from build123d import *

# Parameters (mm, degrees)
SKETCH1_W           = 40
SKETCH1_H           = 33.75
SKETCH1_R           = 2.5
BOSS_EXTRUDE1_DEPTH = 6.25
SKETCH1_3_W         = 40
SKETCH1_3_H         = 6.25
BOSS_EXTRUDE2_DEPTH = 40
FILLET1_R           = 6.25
FILLET2_R           = 1.25
SKETCH2_R           = 5
CUT_EXTRUDE1_DEPTH  = 40


with BuildPart() as part:
    # Sketch1 → Boss-Extrude1 (new body)
    with BuildSketch(Plane(origin=(0, 0, 0), x_dir=(1, 0, 0), z_dir=(0, 1, 0))):
        with Locations((20, 16.875)):
            Rectangle(SKETCH1_W, SKETCH1_H)
        with Locations(Location((10, 15, 0), (0, 0, 270))):
            Circle(SKETCH1_R, mode=Mode.SUBTRACT)
        with Locations(Location((30, 15, 0), (0, 0, 270))):
            Circle(SKETCH1_R, mode=Mode.SUBTRACT)
    extrude(amount=BOSS_EXTRUDE1_DEPTH)

    # Sketch1_3 → Boss-Extrude2 (add)
    with BuildSketch(Plane(origin=(0, 0, 0), x_dir=(1, 0, 0), z_dir=(0, 1, 0))):
        with Locations((20, 36.875)):
            Rectangle(SKETCH1_3_W, SKETCH1_3_H)
    extrude(amount=BOSS_EXTRUDE2_DEPTH)

    # Fillet1
    fillet1_edges = [part.edges().sort_by_distance(p)[0] for p in [
        (20, 0, -40),
    ]]
    fillet(fillet1_edges, radius=FILLET1_R)

    # Fillet2
    fillet2_edges = [part.edges().sort_by_distance(p)[0] for p in [
        (20, 6.25, -33.75),
    ]]
    fillet(fillet2_edges, radius=FILLET2_R)

    # Sketch2 → Cut-Extrude1 (cut)
    with BuildSketch(Plane.XY.offset(-33.75)):
        with Locations((20, 25)):
            Circle(SKETCH2_R)
    extrude(amount=-CUT_EXTRUDE1_DEPTH, mode=Mode.SUBTRACT)


solid = part.part
Can you work these out from the model? Positions are in its coordinate system, mm. A direction names the side the tool comes from. Round coordinates to 2 decimals unless told otherwise and drop trailing zeros. Write each loop counter-clockwise with the first axis right and the second up, starting at its lowest first coordinate (ties: lowest second). Pieces come first, ordered by that corner, then holes. Notation, with made-up numbers: (66.25, 65) -> (91.25, 65) arc R8 cw to (91.25, 79) -> close; hole circle Ø1 at (-26, 57). An arc over 180 degrees is marked (long way). Use one line per item in the form item = value. Start each with the question number.
Q1. Imagine slicing it at D-D (x = 23). Please give me the cut outline in (y, z).
Q2. Which directions (+Z, -Z, +X, -X, +Y, -Y) give clear straight access to the entire face, cutting with the end or side of a thin tool? Please do faces 1 (the face through (18.92, 20.12, -36.83)), 2 (the face through (15, 20, -33.75)).
Q3. Imagine slicing it at A-A (x = 30). Please give me the cut outline in (y, z), then the cut area to 3 significant figures.
Q4. Imagine slicing it at C-C (y = 25). Please give me the cut outline in (x, z), then the cut area to 4 significant figures.
Q5. If I drill on probe 1 along X at (y, z) = (2, -15); probe 2 along Z at (x, y) = (22, 8); probe 3 along Y at (x, z) = (20, -20), over which ranges is the centre line in solid material (lowest first)? Write a range as [from, to].
Q6. Imagine slicing it at B-B (z = -15). Please give me the cut outline in (x, y), then the cut area to 4 significant figures.
Q7. We'd pull the mould along Z, two halves only. Please class faces 3 (the face through (20, 3, 0)), 4 (the face through (31.69, 3.08, -16.84)), 5 (the face through (20, 0, -17)): +Z half, -Z half, draft (parallel to the pull), parting line (faces both ways), or undercut.
Q8. I'm going to push flat-ended pins straight in: P1, Ø12, axis at x = 7, y = 33.5, coming from the +Z side; P2, Ø16, axis at x = 26.5, z = -13, coming from the +Y side; P3, Ø3, axis at x = 31.5, y = 8.5, coming from the +Z side. Where does each tip first touch, or does it pass through?
Worked out:
q1.outline = (0, -33.75) arc R6.25 ccw to (6.25, -40) -> (21, -40) -> (21, -33.75) -> (7.5, -33.75) arc R1.25 cw to (6.25, -32.5) -> (6.25, 0) -> (0, 0) -> close; (29, -40) -> (40, -40) -> (40, -33.75) -> (29, -33.75) -> close
q2.face_1 = +Z, -Z
q2.face_2 = +Z, +X, -X, +Y
q3.outline = (0, -33.75) arc R6.25 ccw to (6.25, -40) -> (40, -40) -> (40, -33.75) -> (7.5, -33.75) arc R1.25 cw to (6.25, -32.5) -> (6.25, -17.5) -> (0, -17.5) -> close; (0, -12.5) -> (6.25, -12.5) -> (6.25, 0) -> (0, 0) -> close
q3.area = 422 mm^2
q4.outline = (0, -40) -> (15, -40) -> (15, -33.75) -> (0, -33.75) -> close; (25, -40) -> (40, -40) -> (40, -33.75) -> (25, -33.75) -> close
q4.area = 187.5 mm^2
q5.probe_1 = [0, 7.5], [12.5, 27.5], [32.5, 40]
q5.probe_2 = [-40, -33.75]
q5.probe_3 = [0, 6.25]
q6.outline = (0, 0) -> (7.5, 0) -> (7.5, 6.25) -> (0, 6.25) -> close; (12.5, 0) -> (27.5, 0) -> (27.5, 6.25) -> (12.5, 6.25) -> close; (32.5, 0) -> (40, 0) -> (40, 6.25) -> (32.5, 6.25) -> close
q6.area = 187.5 mm^2
q7.face_3 = +Z half
q7.face_4 = undercut
q7.face_5 = draft
q8.P1 = -33.75
q8.P2 = 6.25
q8.P3 = -33.65
